Here's how the part is built. I have some questions about the finished solid (model axes, mm). Coordinates: 2 decimals unless noted, no trailing zeros. Loops run counter-clockwise (first coordinate to the right, second up) from the corner with the lowest first, then second, coordinate; pieces in that order, holes last.
```python
from build123d import *

# Parameters (mm, degrees)
F0_W     = 50.8
F0_H     = 50.8
F1_DEPTH = 8
F2_R     = 2
F3_DEPTH = 8


with BuildPart() as f1:
    # F0 (on Top) → F1 (new body)
    with BuildSketch(Plane.XY):
        Rectangle(F0_W, F0_H)
    extrude(amount=F1_DEPTH)

    # F2 (on Top) → F3 (cut, through all)
    with BuildSketch(Plane.XY):
        with Locations((-12.621296, 7.5)):
            Circle(F2_R)
        with Locations((12.621296, 7.5)):
            Circle(F2_R)
    extrude(amount=F3_DEPTH, mode=Mode.SUBTRACT)


solid = f1.part
```
1. I want a section at A-A (y = 7.5). Please give me the cut outline in (x, z), then the cut area to 3 significant figures.
2. I want a section at B-B (x = -11.5). Please give me the cut outline in (y, z), then the cut area to 3 significant figures.
3. We'd pull the mould along X, two halves only. Please class faces 1 (the flat face through (0, -25.4, 4)), 2 (the flat face through (-25.4, 0, 4)), 3 (the cylindrical face through (-10.714, 8.101, 3.944)): +X half, -X half, draft (parallel to the pull), parting line (faces both ways), or undercut.
4. I need wall thicknesses on line 1 along Y through (x, z) = (-12.5, 5); line 2 along X through (y, z) = (6, 1); line 3 along X through (y, z) = (7, 1.25). Which ranges of each line are inside material? Lowest first, please.
Response values:
1. outline: (-25.4, 0) - (-14.62, 0) - (-14.62, 8) - (-25.4, 8) - close; (-10.62, 0) - (10.62, 0) - (10.62, 8) - (-10.62, 8) - close; (14.62, 0) - (25.4, 0) - (25.4, 8) - (14.62, 8) - close
1. area: 342 mm2
2. outline: (-25.4, 0) - (5.84, 0) - (5.84, 8) - (-25.4, 8) - close; (9.16, 0) - (25.4, 0) - (25.4, 8) - (9.16, 8) - close
2. area: 380 mm2
3. face 1: draft
3. face 2: -X half
3. face 3: undercut
4. line 1: y = -25.4 to 5.5, 9.5 to 25.4
4. line 2: x = -25.4 to -13.94, -11.3 to 11.3, 13.94 to 25.4
4. line 3: x = -25.4 to -14.56, -10.68 to 10.68, 14.56 to 25.4
